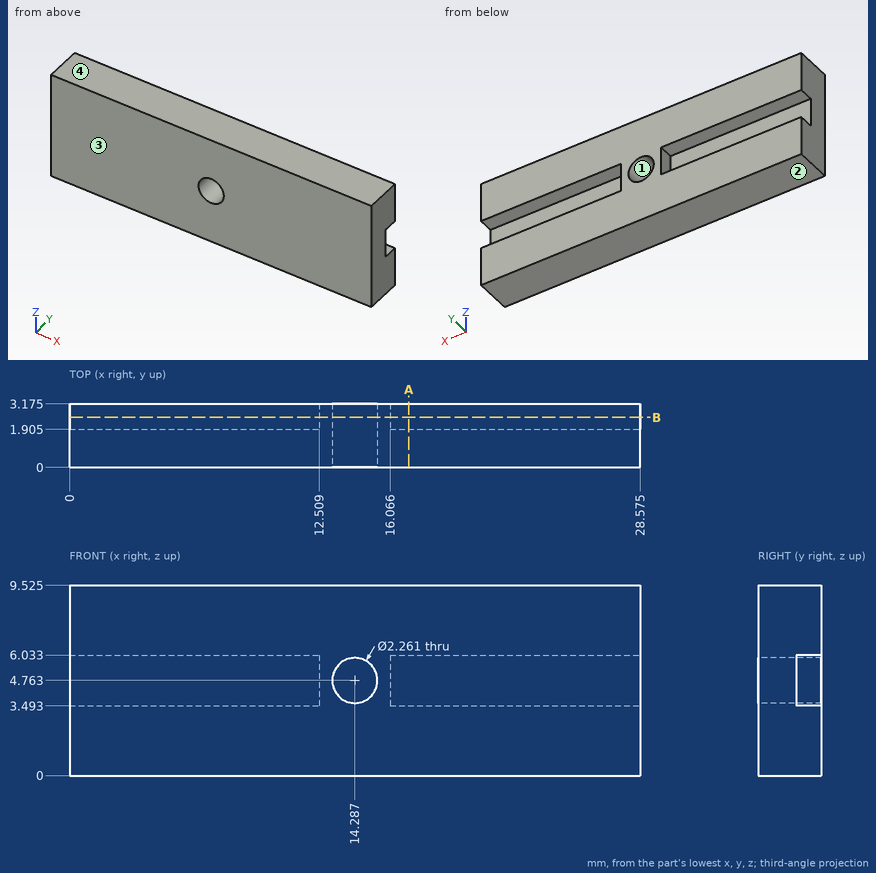
For this review, use the dimensioned drawing (mm, ordinates from the lowest corner) and the shaded views. Round coordinates to 2 decimals unless told otherwise and drop trailing zeros. Order: outer loops, then holes, each group sorted by start corner. A loop starts at its lowest first (then second) coordinate and runs counter-clockwise, first axis right, second up. Notation, with made-up numbers: (6, -2) -> (53, -2) arc R22 cw to (53, 7) -> close; hole circle Ø1 at (-8.75, 56). An arc over 180 degrees is marked (long way). Use CSV: the item, a comma, the result in double quotes. Start each with the question number.
(1) Mouldability with a two-part tool opening along Z and no side actions: class the marked faces 1, 2, 3 and 4 as pulls with the +Z half, pulls with the -Z half, needs draft (parallel to the pull), parting line crosses it, or undercut.
(2) Consider section B-B on y = 2.5. Write out the cut boundary in (x, z) (1 decimal).
(3) Wall thickness on probe 1 along Z at (x, y) = (6.5, 2.7) (1 decimal); probe 2 along Y at (x, z) = (16.5, 6) (1 decimal); probe 3 along X at (y, z) = (1.3, 4) (1 decimal): over which ranges is each line inside the solid? List them lowest first. Write a range as from..to.
(4) Insertion check: pin 1 (2 mm diameter, centred on x = 14.29, z = 4.76, fed in from -Y); pin 2 (0.8 mm diameter, centred on x = 25, z = 5.5, fed in from +Y) (1 decimal). Each pin has a flat end and moves straight along its axis. Give the tip position at first contact, or say it passes through.
(5) Consider section A-A on x = 17. Write out the cut boundary in (y, z) (1 decimal).
Responses:
1,face 1,"undercut"
1,face 2,"pulls with the -Z half"
1,face 3,"needs draft"
1,face 4,"pulls with the +Z half"
2,outline,"(0, 0) -> (28.6, 0) -> (28.6, 3.5) -> (16.1, 3.5) -> (16.1, 6) -> (28.6, 6) -> (28.6, 9.5) -> (0, 9.5) -> (0, 6) -> (12.5, 6) -> (12.5, 3.5) -> (0, 3.5) -> close; hole circle Ø2.3 at (14.3, 4.8)"
3,probe 1,"0..3.5, 6..9.5"
3,probe 2,"0..1.9"
3,probe 3,"0..13.5, 15.1..28.6"
4,pin 1,"through"
4,pin 2,"y = 1.9"
5,outline,"(0, 0) -> (3.2, 0) -> (3.2, 3.5) -> (1.9, 3.5) -> (1.9, 6) -> (3.2, 6) -> (3.2, 9.5) -> (0, 9.5) -> close"
